Geometry: see drawing. Coordinates: mm, zero at the bounding-box minimum. A direction names the side the tool comes from. Coordinates: 2 decimals unless noted, no trailing zeros. Loops run counter-clockwise (first coordinate to the right, second up) from the corner with the lowest first, then second, coordinate; pieces in that order, holes last. Notation, with made-up numbers: (25, 52.25) -> (37, 52.25) arc R19 cw to (37, 58.25) -> close; hole circle Ø2 at (2, -29). An arc over 180 degrees is marked (long way). One line per item, written item: value. Start each with the question number.
Item 1: Section query D-D on y = 42.5. Return loops of the section in (x, z) (1 decimal).
Item 2: Mould query, pull axis X, two halves, no side actions, for the marked faces 4, 5 and 6. Classes: +X half, -X half, draft (parallel to the pull), parting line (faces both ways), or undercut.
Item 3: Ray query, probe 1 along Z at (x, y) = (44, 55.5); probe 2 along Z at (x, y) = (74, 48); probe 3 along X at (y, z) = (21.5, 8) (1 decimal). Return the intervals inside material, ascending. Write a range as from..to.
Item 4: Set-up query: the marked faces 1, 2 and 3. Return all of +Z, -Z, +X, -X, +Y, -Y with unobstructed straight access to the full face (end or side cutting, diameter ignored); none if empty.
Item 5: Section query A-A on y = 21. Return loops of the section in (x, z), then the cut area to 3 significant figures.
Item 6: Contact query for flat-ended pins moving along their axis: pin 1 Ø12 at (y, z) = (39.5, 52) entering from -X; pin 2 Ø1 at (x, y) = (51, 70) entering from -Z; pin 3 Ø1.5 at (y, z) = (31.5, 49) entering from -X; pin 4 Ø1 at (y, z) = (48.5, 11) entering from +X. Output: stop coordinate, or through.
Item 7: Section query C-C on z = 19. Return loops of the section in (x, y).
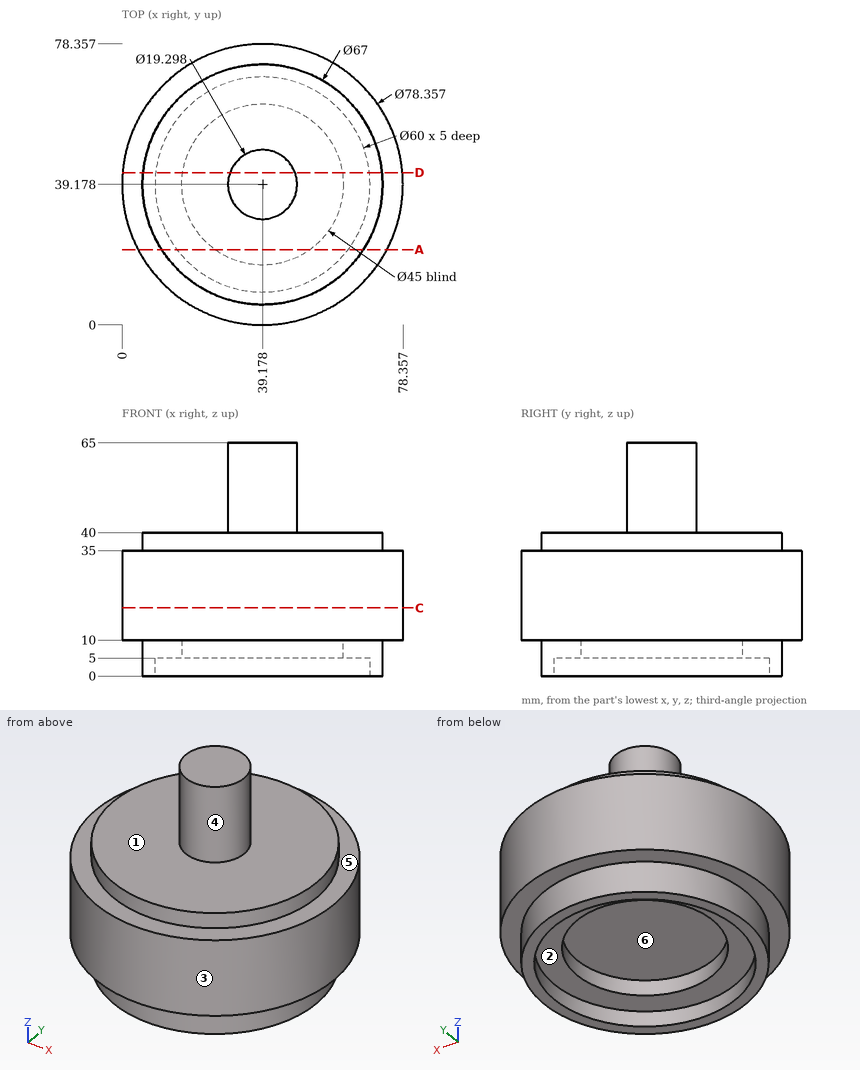
Reply:
1. outline: (0.1, 10) -> (5.8, 10) -> (5.8, 0) -> (9.4, 0) -> (9.4, 5) -> (16.9, 5) -> (16.9, 10) -> (61.4, 10) -> (61.4, 5) -> (69, 5) -> (69, 0) -> (72.5, 0) -> (72.5, 10) -> (78.2, 10) -> (78.2, 35) -> (72.5, 35) -> (72.5, 40) -> (48.2, 40) -> (48.2, 65) -> (30.1, 65) -> (30.1, 40) -> (5.8, 40) -> (5.8, 35) -> (0.1, 35) -> close
2. face 4: parting line
2. face 5: draft
2. face 6: undercut
3. probe 1: z = 10..40
3. probe 2: z = 10..35
3. probe 3: x = 10.7..25.3, 53.1..67.6
4. face 1: +Z
4. face 2: -Z
4. face 3: +Z, -Z
5. outline: (4.47, 10) -> (11.04, 10) -> (11.04, 0) -> (15.31, 0) -> (15.31, 5) -> (25.92, 5) -> (25.92, 10) -> (52.44, 10) -> (52.44, 5) -> (63.04, 5) -> (63.04, 0) -> (67.32, 0) -> (67.32, 10) -> (73.88, 10) -> (73.88, 35) -> (67.32, 35) -> (67.32, 40) -> (11.04, 40) -> (11.04, 35) -> (4.47, 35) -> close
5. area: 2,210 mm²
6. pin 1: stops at x = 29.53
6. pin 2: stops at z = 0
6. pin 3: stops at x = 32.46
6. pin 4: stops at x = 77.35
7. outline: circle Ø78.36 at (39.18, 39.18)
